Model file for the job. Use its own axes, mm. Round coordinates to 2 decimals unless told otherwise and drop trailing zeros. Loops run counter-clockwise (first coordinate to the right, second up) from the corner with the lowest first, then second, coordinate; pieces in that order, holes last. Notation, with made-up numbers: M 79,28.5 L 99,28.5 A18 ccw 99,49.5 Z; hole C 39.5,71.5 d2. An arc over 180 degrees is marked long. Answer in a Markdown table with one row per item.
from build123d import *

# Parameters (mm, degrees)
ESQUISSE1_R        = 45
BOSS_EXTRU_1_DEPTH = 10


with BuildPart() as part:
    # Esquisse1 → Boss.-Extru.1 (new body)
    with BuildSketch(Plane(origin=(0, 0, 0), x_dir=(1, 0, 0), z_dir=(0, 1, 0))):
        with BuildLine():
            Line((0, 0), (0, 600))
            ThreePointArc((0, 600), (150, 750), (300, 600))
            Line((300, 600), (300, 0))
            Line((300, 0), (0, 0))
        make_face()
        with Locations(Location((150, 155, 0), (0, 0, 270))):
            Circle(ESQUISSE1_R, mode=Mode.SUBTRACT)
        with Locations(Location((150, 265, 0), (0, 0, 270))):
            Circle(ESQUISSE1_R, mode=Mode.SUBTRACT)
        with Locations(Location((150, 375, 0), (0, 0, 270))):
            Circle(ESQUISSE1_R, mode=Mode.SUBTRACT)
        with Locations(Location((150, 485, 0), (0, 0, 270))):
            Circle(ESQUISSE1_R, mode=Mode.SUBTRACT)
        with Locations(Location((150, 595, 0), (0, 0, 270))):
            Circle(ESQUISSE1_R, mode=Mode.SUBTRACT)
    extrude(amount=BOSS_EXTRU_1_DEPTH)


solid = part.part
1. Mould opens along X. For faces 1 (the cylindrical face through (146.702, 4.93, -749.964)), 2 (the cylindrical face through (163.52, 4.93, -442.08)), 3 (the flat face through (85, 10, -380)), 4 (the cylindrical face through (163.52, 4.93, -552.08)) say: +X half, -X half, draft (parallel to the pull), parting line (faces both ways), or undercut.
Verdict:
| item | result |
|---|---|
| face 1 | parting line |
| face 2 | undercut |
| face 3 | draft |
| face 4 | undercut |
2. Saw through at A-A (x = 150). Write the cut outline in (y, z), and give its area (3 significant figures).
Verdict:
| item | result |
|---|---|
| outline | M 0,-750 L 10,-750 L 10,-640 L 0,-640 Z; M 0,-550 L 10,-550 L 10,-530 L 0,-530 Z; M 0,-440 L 10,-440 L 10,-420 L 0,-420 Z; M 0,-330 L 10,-330 L 10,-310 L 0,-310 Z; M 0,-220 L 10,-220 L 10,-200 L 0,-200 Z; M 0,-110 L 10,-110 L 10,0 L 0,0 Z |
| area | 3,000 mm² |
3. Saw through at B-B (z = -119). Write the cut outline in (x, y), and give its area (3 significant figures).
Verdict:
| item | result |
|---|---|
| outline | M 0,0 L 123,0 L 123,10 L 0,10 Z; M 177,0 L 300,0 L 300,10 L 177,10 Z |
| area | 2,460 mm² |
4. Pin check, flat tips, straight feed: pin 1 (1.5 mm diameter, centred on x = 133, z = -216, fed in from -Y); pin 2 (5 mm diameter, centred on x = 265.5, y = 2, fed in from -Z); pin 3 (2 mm diameter, centred on x = 97, y = 8.5, fed in from -Z). Stop position of each tip, or through.
Verdict:
| item | result |
|---|---|
| pin 1 | stops at y = 0 |
| pin 2 | stops at z = -698.65 |
| pin 3 | stops at z = -740.7 |
5. Saw through at D-D (z = -375). Write the cut outline in (x, y), and give its area (3 significant figures).
Verdict:
| item | result |
|---|---|
| outline | M 0,0 L 105,0 L 105,10 L 0,10 Z; M 195,0 L 300,0 L 300,10 L 195,10 Z |
| area | 2,100 mm² |
6. Saw through at C-C (y = 7.25). Write the cut outline in (x, z).
Verdict:
| item | result |
|---|---|
| outline | M 0,-600 A150 ccw 300,-600 L 300,0 L 0,0 Z; hole C 150,-595 d90; hole C 150,-485 d90; hole C 150,-375 d90; hole C 150,-265 d90; hole C 150,-155 d90 |
7. Wall check: probe 1 along Z at (x, y) = (163.5, 7.5); probe 2 along X at (y, z) = (5, -155); probe 3 along Z at (x, y) = (109, 1.25). Give the ranges that are in metal, low to high.
Verdict:
| item | result |
|---|---|
| probe 1 | z = -749.39 to -637.93, -552.07 to -527.93, -442.07 to -417.93, -332.07 to -307.93, -222.07 to -197.93, -112.07 to 0 |
| probe 2 | x = 0 to 105, 195 to 300 |
| probe 3 | z = -744.29 to -613.55, -576.45 to -503.55, -466.45 to -393.55, -356.45 to -283.55, -246.45 to -173.55, -136.45 to 0 |
